from build123d import *

# Parameters (mm, degrees)
F0_R          = 12.7
F0_R_2        = 10.16
F1_DEPTH      = 2.54
F1_DEPTH_BACK = 2.54
F2_R          = 1.016


with BuildPart() as f1:
    # F0 (on Top) → F1 (new body, two sides)
    with BuildSketch(Plane.XY) as f1_sk:
        Circle(F0_R)
        Circle(F0_R_2, mode=Mode.SUBTRACT)
    extrude(amount=F1_DEPTH)
    extrude(f1_sk.sketch, amount=-F1_DEPTH_BACK)

    # F2
    f2_edges = [f1.edges().sort_by_distance(p)[0] for p in [
        (12.7, 0, -1.27),
        (-12.7, 0, 0),
        (-12.7, 0, -2.54),
        (10.16, 0, -1.27),
        (-10.16, 0, 0),
        (-10.16, 0, -2.54),
        (-12.7, 0, 2.54),
        (-10.16, 0, 2.54),
    ]]
    fillet(f2_edges, radius=F2_R)


solid = f1.part
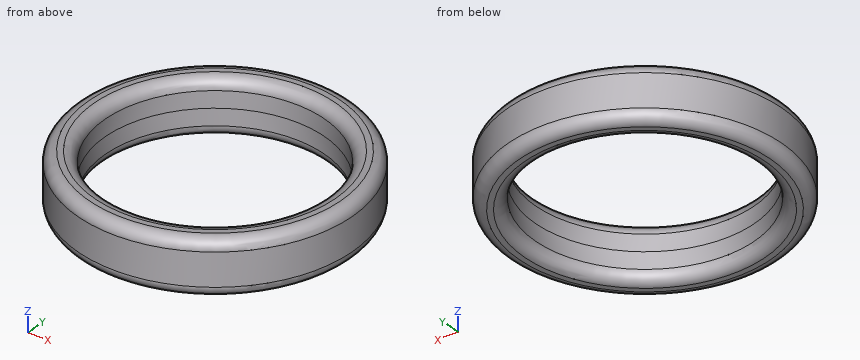
Could you check a few things on this model? Use its own coordinates, in mm. Give positions to 0.01 mm unless a question says otherwise; leave off trailing zeros. Order: outer loops, then holes, each group sorted by start corner. A loop starts at its lowest first (then second) coordinate and runs counter-clockwise, first axis right, second up.
1. I need wall thicknesses on L1, parallel to Y at x = 0, z = -0.85; L2, parallel to Y at x = 4.25, z = 1.2; L3, parallel to X at y = 1.5, z = -0.65. Which ranges of each line are inside material? Lowest first, please.
Answers below:
L1: y = -12.7 to -10.16, 10.16 to 12.7
L2: y = -11.97 to -9.23, 9.23 to 11.97
L3: x = -12.61 to -10.05, 10.05 to 12.61
2. Suppose I cut it at C-C (z = 0.75). Write out the boundary of the cut face in (x, y).
Answers below:
outline: circle Ø25.4 at (0, 0); hole circle Ø20.32 at (0, 0)
3. Suppose I cut it at A-A (x = 0). Write out the boundary of the cut face in (y, z), plus the area to 3 significant figures.
Answers below:
outline: (-12.7, -1.52) arc R1.02 ccw to (-11.68, -2.54) - (-11.18, -2.54) arc R1.02 ccw to (-10.16, -1.52) - (-10.16, 1.52) arc R1.02 ccw to (-11.18, 2.54) - (-11.68, 2.54) arc R1.02 ccw to (-12.7, 1.52) - close; (10.16, -1.52) arc R1.02 ccw to (11.18, -2.54) - (11.68, -2.54) arc R1.02 ccw to (12.7, -1.52) - (12.7, 1.52) arc R1.02 ccw to (11.68, 2.54) - (11.18, 2.54) arc R1.02 ccw to (10.16, 1.52) - close
area: 24.0 mm2
4. Suppose I cut it at D-D (z = -1.95). Write out the boundary of the cut face in (x, y).
Answers below:
outline: circle Ø25.21 at (0, 0); hole circle Ø20.51 at (0, 0)
5. For pin 1 (3 mm diameter, centred on y = -2.5, z = -0.5, fed in from -X); pin 2 (3 mm diameter, centred on x = 7, y = 5.5, fed in from -Z); pin 3 (3 mm diameter, centred on y = -7.5, z = -1, fed in from -X); pin 4 (3 mm diameter, centred on x = 0.5, z = 0, fed in from +Y), each with a flat end and sliding along its axis, tell me the tip position at first contact or that it passes through.
Answers below:
pin 1: stops at x = -12.66
pin 2: stops at z = -2.18
pin 3: stops at x = -11.19
pin 4: stops at y = 12.7
